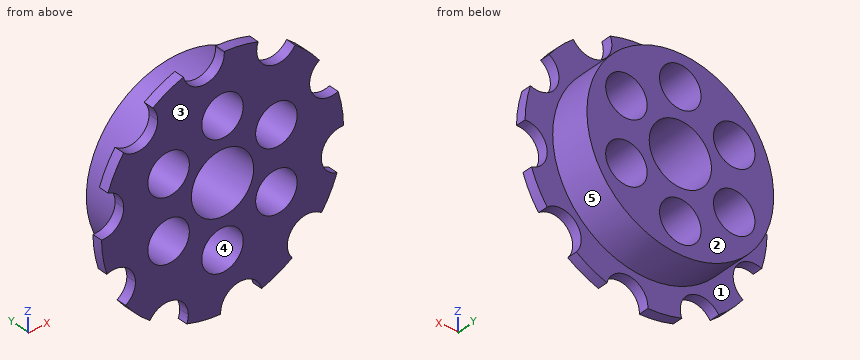
from build123d import *

# Parameters (mm, degrees)
F0_R     = 27
F1_DEPTH = 15
F2_R     = 35
F2_R_2   = 27
F3_DEPTH = 3
F4_R     = 9
F5_DEPTH = 15.001
F6_R     = 6
F7_DEPTH = 15.001


with BuildPart() as f1:
    # F0 (on Front) → F1 (new body)
    with BuildSketch(Plane.XZ):
        Circle(F0_R)
    extrude(amount=-F1_DEPTH)

    # F2 (on face) → F3 (join)
    with BuildSketch(Plane.XZ):
        Circle(F2_R)
        Circle(F2_R_2, mode=Mode.SUBTRACT)
    extrude(amount=-F3_DEPTH)

    # F4 (on face) → F5 (cut, through all)
    with BuildSketch(Plane.XZ):
        Circle(F4_R)
    extrude(amount=-F5_DEPTH, mode=Mode.SUBTRACT)

    # F6 (on face) → F7 (cut, through all)
    with BuildSketch(Plane.XZ):
        with Locations((0, 18)):
            Circle(F6_R)
        with Locations((-15.5884572681, 9)):
            Circle(F6_R)
        with Locations((-15.5884572681, -9)):
            Circle(F6_R)
        with Locations((0, -18)):
            Circle(F6_R)
        with BuildLine():
            ThreePointArc((-28.6121091704, 20.1580556806), (-22.2169623686, 19.3090576187), (-18.7487373415, 24.7487373415))
            ThreePointArc((-18.7487373415, 24.7487373415), (-19.1120676703, 26.8049365092), (-20.1580556806, 28.6121091704))
            ThreePointArc((-20.1580556806, 28.6121091704), (-24.7487373415, 24.7487373415), (-28.6121091704, 20.1580556806))
        make_face()
        with BuildLine():
            ThreePointArc((0.5095661882, 34.9962904077), (-5.4752062764, 34.5690919208), (-11.2990747198, 33.1259854265))
            ThreePointArc((-11.2990747198, 33.1259854265), (-4.7482986689, 28.6132875813), (0.5247937236, 34.5690919208))
            ThreePointArc((0.5247937236, 34.5690919208), (0.5209856313, 34.782826818), (0.5095661882, 34.9962904077))
        make_face()
        with BuildLine():
            ThreePointArc((-34.9962904077, -0.5095661882), (-34.5690919208, 5.4752062764), (-33.1259854265, 11.2990747198))
            ThreePointArc((-33.1259854265, 11.2990747198), (-40.4952219644, 6.4138130666), (-34.9962904077, -0.5095661882))
        make_face()
        with BuildLine():
            ThreePointArc((-28.5690919208, 5.4752062764), (-29.8437009864, 9.1725946137), (-33.1259854265, 11.2990747198))
            ThreePointArc((-33.1259854265, 11.2990747198), (-34.5690919208, 5.4752062764), (-34.9962904077, -0.5095661882))
            ThreePointArc((-34.9962904077, -0.5095661882), (-30.4802773568, 1.084124922), (-28.5690919208, 5.4752062764))
        make_face()
        with BuildLine():
            ThreePointArc((20.9825510926, 28.0130781894), (15.8896674909, 31.1852283466), (10.3298222323, 33.4409146503))
            ThreePointArc((10.3298222323, 33.4409146503), (13.1657244924, 25.8391892015), (20.9825510926, 28.0130781894))
        make_face()
        with BuildLine():
            ThreePointArc((-25.1852283466, -15.8896674909), (-27.8336703374, -10.9130161156), (-33.4409146503, -10.3298222323))
            ThreePointArc((-33.4409146503, -10.3298222323), (-31.1852283466, -15.8896674909), (-28.0130781894, -20.9825510926))
            ThreePointArc((-28.0130781894, -20.9825510926), (-25.9396158493, -18.8023208394), (-25.1852283466, -15.8896674909))
        make_face()
        with BuildLine():
            ThreePointArc((33.4409146503, 10.3298222323), (31.1852283466, 15.8896674909), (28.0130781894, 20.9825510926))
            ThreePointArc((28.0130781894, 20.9825510926), (25.8391892015, 13.1657244924), (33.4409146503, 10.3298222323))
        make_face()
        with BuildLine():
            ThreePointArc((37.1852283466, 15.8896674909), (34.0978816951, 21.1352799882), (28.0130781894, 20.9825510926))
            ThreePointArc((28.0130781894, 20.9825510926), (31.1852283466, 15.8896674909), (33.4409146503, 10.3298222323))
            ThreePointArc((33.4409146503, 10.3298222323), (36.1618797219, 12.5381094817), (37.1852283466, 15.8896674909))
        make_face()
        with BuildLine():
            ThreePointArc((-9.8896674909, -31.1852283466), (-14.2400162566, -25.4164632443), (-20.9825510926, -28.0130781894))
            ThreePointArc((-20.9825510926, -28.0130781894), (-15.8896674909, -31.1852283466), (-10.3298222323, -33.4409146503))
            ThreePointArc((-10.3298222323, -33.4409146503), (-10.00073416, -32.3343428858), (-9.8896674909, -31.1852283466))
        make_face()
        with BuildLine():
            ThreePointArc((35, 0), (34.9990725896, 0.2547898454), (34.9962904077, 0.5095661882))
            ThreePointArc((34.9962904077, 0.5095661882), (28.6429618773, -4.5365994862), (33.1259854265, -11.2990747198))
            ThreePointArc((33.1259854265, -11.2990747198), (34.5283180153, -5.726714157), (35, 0))
        make_face()
        with BuildLine():
            ThreePointArc((40.5690919208, -5.4752062764), (38.9601732752, -1.3863917123), (34.9962904077, 0.5095661882))
            ThreePointArc((34.9962904077, 0.5095661882), (34.9990725896, 0.2547898454), (35, 0))
            ThreePointArc((35, 0), (34.5283180153, -5.726714157), (33.1259854265, -11.2990747198))
            ThreePointArc((33.1259854265, -11.2990747198), (38.2664802582, -10.2005972108), (40.5690919208, -5.4752062764))
        make_face()
        with BuildLine():
            ThreePointArc((11.2990747198, -33.1259854265), (4.5365994862, -28.6429618773), (-0.5095661882, -34.9962904077))
            ThreePointArc((-0.5095661882, -34.9962904077), (5.4752062764, -34.5690919208), (11.2990747198, -33.1259854265))
        make_face()
        with BuildLine():
            ThreePointArc((20.1580556806, -28.6121091704), (24.7487373415, -24.7487373415), (28.6121091704, -20.1580556806))
            ThreePointArc((28.6121091704, -20.1580556806), (20.5060966544, -20.5060966544), (20.1580556806, -28.6121091704))
        make_face()
        with Locations((15.5884572681, -9)):
            Circle(F6_R)
        with Locations((15.5884572681, 9)):
            Circle(F6_R)
    extrude(amount=-F7_DEPTH, mode=Mode.SUBTRACT)


solid = f1.part
Geometry check sheet. Reference: the model listing, model coordinates, mm. Face numbers are marked on the shaded views. A direction names the side the tool comes from. Give positions to 0.01 mm unless a question says otherwise; leave off trailing zeros. Write each loop counter-clockwise with the first axis right and the second up, starting at its lowest first coordinate (ties: lowest second). Pieces come first, ordered by that corner, then holes.
1) Cross-section at C-C (z = -4). Record the boundary of the cut face in (x, y), plus the area to 3 significant figures.
Values follow:
outline: (-34.77, 0) - (-18.91, 0) - (-18.91, 15) - (-26.7, 15) - (-26.7, 3) - (-34.77, 3) - close; (-12.27, 0) - (-8.06, 0) - (-8.06, 15) - (-12.27, 15) - close; (8.06, 0) - (12.27, 0) - (12.27, 15) - (8.06, 15) - close; (18.91, 0) - (28.75, 0) - (28.75, 3) - (26.7, 3) - (26.7, 15) - (18.91, 15) - close
area: 391 mm2
2) Set-up check for the marked faces 1 and 2: record each of +Z, -Z, +X, -X, +Y, -Y from which the full face is reachable in a straight line by a thin tool's end or side.
Values follow:
face 1: +Y
face 2: +Z, -Z, +X, -X, +Y
3) Cross-section at B-B (x = 7.5). Record the boundary of the cut face in (y, z), plus the area to 3 significant figures.
Values follow:
outline: (0, -28.92) - (3, -28.92) - (3, -25.94) - (15, -25.94) - (15, -4.97) - (0, -4.97) - close; (0, 4.97) - (15, 4.97) - (15, 25.94) - (3, 25.94) - (3, 34.19) - (0, 34.19) - close
area: 663 mm2
4) Go/stop test with flat-tipped pins: pin 1 Ø5 at (x, y) = (-23.5, 12.5) entering from -Z; pin 2 Ø7 at (x, z) = (0, 18) entering from -Y; pin 3 Ø1 at (y, z) = (6, -11.5) entering from +X; pin 4 Ø2 at (x, y) = (-13.5, 13) entering from -Z. Record where each tip stops, or that it passes through.
Values follow:
pin 1: stops at z = -16.97
pin 2: passes through
pin 3: stops at x = 24.66
pin 4: stops at z = -23.93
5) Release check for a two-part mould opening along Z. For the marked faces 3, 4 and 5 record: released by +Z, released by -Z, zero draft, split by the parting line, or undercut.
Values follow:
face 3: zero draft
face 4: undercut
face 5: split by the parting line
6) Thickness scan on line 1 (Z direction, x = 0, y = 4.25); line 2 (Z direction, x = 14, y = 0.75); line 3 (X direction, y = 2.5, z = -10.5). Record the ranges inside material, lowest first.
Values follow:
line 1: z = -27 to -24, -12 to -9, 9 to 12, 24 to 27
line 2: z = -32.08 to -14.79, -3.21 to 3.21, 14.79 to 25.49
line 3: x = -28.55 to -21.4, -9.78 to 9.78, 21.4 to 31.29
7) Cross-section at D-D (x = 22.5). Record the boundary of the cut face in (y, z), plus the area to 3 significant figures.
Values follow:
outline: (0, -19.19) - (3, -19.19) - (3, -14.92) - (15, -14.92) - (15, 14.92) - (3, 14.92) - (3, 26.81) - (0, 26.81) - close
area: 496 mm2
8) Cross-section at A-A (y = 11.75). Record the boundary of the cut face in (x, z).
Values follow:
outline: circle Ø54 at (0, 0); hole circle Ø12 at (-15.59, -9); hole circle Ø12 at (-15.59, 9); hole circle Ø18 at (0, 0); hole circle Ø12 at (0, -18); hole circle Ø12 at (0, 18); hole circle Ø12 at (15.59, -9); hole circle Ø12 at (15.59, 9)
